Design review of the part built by this model. Coordinates are the model's own, in mm. Coordinates: 2 decimals unless noted, no trailing zeros. Loops run counter-clockwise (first coordinate to the right, second up) from the corner with the lowest first, then second, coordinate; pieces in that order, holes last. Notation, with made-up numbers: (73, 11) -> (89, 11) arc R18 cw to (89, 17) -> close; hole circle Ø5 at (-28.75, 89). An arc over 180 degrees is marked (long way). Answer as a JSON object with one key per item and string values.
Autodesk Inventor part; units mm, degrees
ref_plane "1_XY" through (0, 0, 0) normal (0, 0, 1) x (1, 0, 0)
ref_plane "1_YZ" through (0, 0, 0) normal (1, 0, 0) x (0, 1, 0)
ref_plane "1_ZX" through (0, 0, 0) normal (0, 1, 0) x (0, 0, 1)
sketch "Sketch_1" plane through (0, 0, 0) normal (0, 0, 1) x (1, 0, 0)
  line L0 (-4.5, 4.5) -> (-4.5, -4.5)
  line L1 (-4.5, -4.5) -> (4.5, -4.5)
  line L2 (4.5, -4.5) -> (4.5, 4.5)
  line L3 (4.5, 4.5) -> (-4.5, 4.5)
extrude "Extrusion1" add sketch "Sketch_1" against normal blind 3
sketch "Sketch_2" plane through (0, 0, 0) normal (1, 0, 0) x (0, 1, 0)
  line L0 (0, -3) -> (0, 0)
  line L1 (0, 0) -> (2.5, 0)
  line L2 (2.5, 0) -> (2.067, -0.433)
  line L3 (2.067, -0.433) -> (2.067, -2.567)
  line L4 (2.067, -2.567) -> (2.5, -3)
  line L5 (2.5, -3) -> (0, -3)
  line L6 (0, -3) -> (0, 0)
revolve "Revolution1" cut sketch "Sketch_2" angle 360 about axis through (0, 0, -3) along (0, 0, -1)
thread "Thread1"
ref_plane "1_XY" through (0, 0, 0) normal (0, 0, 1) x (1, 0, 0)
ref_plane "1_YZ" through (0, 0, 0) normal (1, 0, 0) x (0, 1, 0)
ref_plane "1_ZX" through (0, 0, 0) normal (0, 1, 0) x (0, 0, 1)
properties part number "14122"
1) Wall thickness on probe 1 along X at (y, z) = (0, -1.4); probe 2 along Y at (x, z) = (-0.5, -1.8); probe 3 along Y at (x, z) = (0.25, -1.05): over which ranges is each line inside the solid? List them lowest first.
Completed:
{"probe 1": "-4.5 to -2.07, 2.07 to 4.5", "probe 2": "-4.5 to -2.01, 2.01 to 4.5", "probe 3": "-4.5 to -2.05, 2.05 to 4.5"}
2) The part is to be moulded in two halves that separate along Y. For faces 1 (the flat face through (0, -4.5, -1)), 2 (the cylindrical face through (-1.26, -1.64, -1.51)), 3 (the flat face through (4.5, 0, -1)), say which applies: pulls with the +Y half, pulls with the -Y half, needs draft (parallel to the pull), parting line crosses it, or undercut.
Completed:
{"face 1": "pulls with the -Y half", "face 2": "undercut", "face 3": "needs draft"}
3) Add section C-C, the plane z = -0.85. Give the boundary of the cut face in (x, y), and give its area (3 significant figures).
Completed:
{"outline": "(-4.5, -4.5) -> (4.5, -4.5) -> (4.5, 4.5) -> (-4.5, 4.5) -> close; hole circle Ø4.13 at (0, 0)", "area": "67.6 mm²"}
4) Add section A-A, the plane y = 0. Give the boundary of the cut face in (x, z).
Completed:
{"outline": "(-4.5, -3) -> (-2.5, -3) -> (-2.07, -2.57) -> (-2.07, -0.43) -> (-2.5, 0) -> (-4.5, 0) -> close; (2.07, -2.57) -> (2.5, -3) -> (4.5, -3) -> (4.5, 0) -> (2.5, 0) -> (2.07, -0.43) -> close"}
5) Clearance check with a flat-ended pin moving along its axis: pin 1 Ø2 at (x, y) = (-0.5, 1) entering from +Z. State where the tip first meets the part, or that it passes through.
Completed:
{"pin 1": "z = -0.38"}
